The model under review builds one solid part; all positions refer to its coordinate system, in mm. A direction names the side the tool comes from. Round coordinates to 2 decimals unless told otherwise and drop trailing zeros. Loops run counter-clockwise (first coordinate to the right, second up) from the corner with the lowest first, then second, coordinate; pieces in that order, holes last. Notation, with made-up numbers: (10, 69.25) - (52, 69.25) arc R15 ccw to (52, 87.25) - close; hole circle Ø10 at (22, 47.25). An arc over 180 degrees is marked (long way). Answer as CSV lines item,"result".
from build123d import *

# Parameters (mm, degrees)
F0_W     = 550
F0_H     = 300
F0_R     = 100
F1_DEPTH = 700
F2_W     = 350
F2_H     = 300
F3_ANGLE = 180
F5_D     = 100
F5_DEPTH = 350
F5_TIP   = 30.0430309514
F6_D     = 200
F6_DEPTH = 100
F6_TIP   = 60.0860619028
F7_R     = 150
F8_DEPTH = 300


with BuildPart() as f1:
    # F0 (on Front) → F1 (new body)
    with BuildSketch(Plane.XZ):
        with Locations((275, 150)):
            Rectangle(F0_W, F0_H)
        with Locations((350, 150)):
            Circle(F0_R, mode=Mode.SUBTRACT)
    extrude(amount=F1_DEPTH)

    # F2 (on face) → F3 (revolve)
    with BuildSketch(Plane.YZ.offset(550)):
        with Locations((-525, 150)):
            Rectangle(F2_W, F2_H)
    revolve(axis=Axis((550, -350, 150), (0, 0, 1)), revolution_arc=F3_ANGLE)

    # F5
    with Locations(Plane(origin=(0, 0, 0), x_dir=(0, -1, 0), z_dir=(-1, 0, 0))):
        with Locations((350, 150)):
            Hole(F5_D / 2, depth=F5_DEPTH)
            with Locations((0, 0, -(F5_DEPTH + F5_TIP / 2))):  # 118° drill point
                Cone(0, F5_D / 2, F5_TIP, mode=Mode.SUBTRACT)

    # F6
    with Locations(Plane(origin=(0, 0, 0), x_dir=(0, -1, 0), z_dir=(-1, 0, 0))):
        with Locations((350, 150)):
            Hole(F6_D / 2, depth=F6_DEPTH)
            with Locations((0, 0, -(F6_DEPTH + F6_TIP / 2))):  # 118° drill point
                Cone(0, F6_D / 2, F6_TIP, mode=Mode.SUBTRACT)

    # F7 (on face) → F8 (join)
    with BuildSketch(Plane.XY.offset(300)):
        with Locations((350, -350)):
            Circle(F7_R)
    extrude(amount=F8_DEPTH)


solid = f1.part
1. Take a section at D-D (x = 220). State the section outline as (y, z) points.
Numbers:
outline,"(-700, 0) - (0, 0) - (0, 300) - (-275.17, 300) - (-275.17, 600) - (-424.83, 600) - (-424.83, 300) - (-700, 300) - close; hole circle Ø100 at (-350, 150)"
2. Take a section at B-B (y = -350). State the section outline as (x, z) points, plus the area to 3 significant figures.
Numbers:
outline,"(0, 0) - (900, 0) - (900, 300) - (500, 300) - (500, 600) - (200, 600) - (200, 300) - (0, 300) - (0, 250) - (100, 250) - (130.04, 200) - (263.4, 200) arc R100 cw (long way) to (263.4, 100) - (130.04, 100) - (100, 50) - (0, 50) - close"
area,"292,000 mm²"
3. Clearance check with flat-ended pins moving along their axes: pin 1 (5 mm diameter, centred on x = 226, y = -245, fed in from -Z); pin 2 (10 mm diameter, centred on x = 777.5, y = -124.5, fed in from +Z); pin 3 (10 mm diameter, centred on x = 696.5, z = 75.5, fed in from +Y); pin 4 (2 mm diameter, centred on y = -239.5, z = 466.5, fed in from -X). State where each tip first meets the part, or that it passes through.
Numbers:
pin 1,"stops at z = 0"
pin 2,"stops at z = 300"
pin 3,"stops at y = -29.88"
pin 4,"stops at x = 247.48"
4. Take a section at A-A (x = 350). State the section outline as (y, z) points.
Numbers:
outline,"(-700, 0) - (0, 0) - (0, 50) - (-700, 50) - close; (-700, 250) - (0, 250) - (0, 300) - (-200, 300) - (-200, 600) - (-500, 600) - (-500, 300) - (-700, 300) - close"
5. Take a section at C-C (y = -67.5). State the section outline as (x, z) points.
Numbers:
outline,"(0, 0) - (756.62, 0) - (756.62, 300) - (0, 300) - close; hole circle Ø200 at (350, 150)"
6. Tool access review of faces 4 (the face through (50.7, -429.357, 89.152)), 5 (the face through (456, -345, 0)): name each direction out of +Z, -Z, +X, -X, +Y, -Y from which nothing blocks a thin tool from reaching the whole face with its end or side.
Numbers:
face 4,"-X"
face 5,"-Z, +X, -X, +Y, -Y"
7. Draft analysis for pull direction Y (two halves, no side actions). For faces 1 (the face through (197.654, -303.813, 130.85)), 2 (the face through (430.64, -223.52, 447.9)), 3 (the face through (348, -348, 600)), state which applies: +Y half, -Y half, draft (parallel to the pull), parting line (faces both ways), or undercut.
Numbers:
face 1,"undercut"
face 2,"parting line"
face 3,"draft"
8. Wall thickness on probe 1 along Y at (x, z) = (231, 150); probe 2 along Z at (x, y) = (24, -350); probe 3 along Z at (x, y) = (209, -350): over which ranges is each line inside the solid? List them lowest first.
Numbers:
probe 1,"y = -700 to -400, -300 to 0"
probe 2,"z = 0 to 50, 250 to 300"
probe 3,"z = 0 to 100, 200 to 600"
